Read the model definition and answer for the solid it produces. Units are mm, in the model's axes. A direction names the side the tool comes from. Round coordinates to 2 decimals unless told otherwise and drop trailing zeros. Write each loop counter-clockwise with the first axis right and the second up, starting at its lowest first coordinate (ties: lowest second). Pieces come first, ordered by that corner, then holes.
from build123d import *

# Parameters (mm, degrees)
SKETCH_1_R          = 3.05
EXTRUDE_1_DEPTH     = 12
SKETCH_2_R          = 3.098235282
EXTRUDE_2_DEPTH     = 2
EXTRUDE_3_DEPTH     = 7
CHAMFER_1_SIZE      = 1
SKETCH_6_R          = 3.05
CUT_EXTRUDE_2_DEPTH = 7
SKETCH_7_R          = 3.05
SKETCH_7_R_2        = 3
EXTRUDE_4_DEPTH     = 10
SKETCH_8_R          = 3
EXTRUDE_5_DEPTH     = 1


with BuildPart() as part:
    # 草图1 → 凸台-拉伸1 (new body)
    with BuildSketch(Plane.XY):
        Polygon((1.45714262, 6.138188374), (-2.429083459, 5.822385651), (-5.387482218, 3.282629506), (-6.288045884, -0.510979538), (-4.786789744, -4.109411766), (-1.45714262, -6.138188374), (2.429083459, -5.822385651), (5.387482218, -3.282629506), (6.288045884, 0.510979538), (4.786789744, 4.109411766), align=None)
        Circle(SKETCH_1_R, mode=Mode.SUBTRACT)
    extrude(amount=EXTRUDE_1_DEPTH)

    # 草图2 → 凸台-拉伸2 (add)
    with BuildSketch(Plane.XY.offset(12)):
        Circle(SKETCH_2_R)
    extrude(amount=-EXTRUDE_2_DEPTH)

    # 草图3 → 凸台-拉伸3 (add)
    with BuildSketch(Plane(origin=(0, 0, 10), x_dir=(-1, 0, 0), z_dir=(0, 0, -1))):
        with BuildLine():
            Line((1.45, 2.683281573), (1.45, -2.683281573))
            ThreePointArc((1.45, -2.683281573), (3.05, 0), (1.45, 2.683281573))
        make_face()
    extrude(amount=EXTRUDE_3_DEPTH)

    # 倒角1
    chamfer_1_edges = [part.edges().sort_by_distance(p)[0] for p in [
        (-3.908282839, 4.552507579, 12),
        (-5.837764051, 1.385824984, 12),
        (-5.537417814, -2.310195652, 12),
        (-3.121966182, -5.12380007, 12),
        (0.48597042, -5.980287012, 12),
        (3.908282839, -4.552507579, 12),
        (5.837764051, -1.385824984, 12),
        (5.537417814, 2.310195652, 12),
        (3.121966182, 5.12380007, 12),
        (-0.48597042, 5.980287012, 12),
    ]]
    chamfer(chamfer_1_edges, length=CHAMFER_1_SIZE)

    # 草图5 → 切除-放样1 section 0
    with BuildSketch(Plane.XY.offset(12)):
        Polygon((0.910714137, 3.836367733), (-1.518177162, 3.638991032), (-3.367176386, 2.051643441), (-3.930028677, -0.319362211), (-2.99174359, -2.568382354), (-0.910714137, -3.836367733), (1.518177162, -3.638991032), (3.367176386, -2.051643441), (3.930028677, 0.319362211), (2.99174359, 2.568382354), align=None)
    # 草图4 → 切除-放样1 section 1
    with BuildSketch(Plane.XY.offset(11)):
        Polygon((0.72857131, 3.069094187), (-1.21454173, 2.911192826), (-2.693741109, 1.641314753), (-3.144022942, -0.255489769), (-2.393394872, -2.054705883), (-0.72857131, -3.069094187), (1.21454173, -2.911192826), (2.693741109, -1.641314753), (3.144022942, 0.255489769), (2.393394872, 2.054705883), align=None)
    loft(mode=Mode.SUBTRACT)

    # 草图6 → 切除-拉伸2 (cut)
    with BuildSketch(Plane(origin=(0, 0, 3), x_dir=(-1, 0, 0), z_dir=(0, 0, -1))):
        Circle(SKETCH_6_R)
    extrude(amount=-CUT_EXTRUDE_2_DEPTH, mode=Mode.SUBTRACT)

    # 草图7 → 凸台-拉伸4 (add)
    with BuildSketch(Plane(origin=(0, 0, 0), x_dir=(-1, 0, 0), z_dir=(0, 0, -1))):
        Circle(SKETCH_7_R)
        Circle(SKETCH_7_R_2, mode=Mode.SUBTRACT)
    extrude(amount=-EXTRUDE_4_DEPTH)

    # 草图8 → 凸台-拉伸5 (add)
    with BuildSketch(Plane(origin=(0, 0, 0), x_dir=(-1, 0, 0), z_dir=(0, 0, -1))):
        Polygon((2.429083459, 5.822385651), (-1.45714262, 6.138188374), (-4.786789744, 4.109411766), (-6.288045884, 0.510979538), (-5.387482218, -3.282629506), (-2.429083459, -5.822385651), (1.45714262, -6.138188374), (4.786789744, -4.109411766), (6.288045884, -0.510979538), (5.387482218, 3.282629506), align=None)
        Circle(SKETCH_8_R, mode=Mode.SUBTRACT)
    extrude(amount=EXTRUDE_5_DEPTH)


solid = part.part
Q1. Determine the mould class of faces 3 (the cylindrical face through (3, 0, 5)), 4 (the flat face through (5.844, -1.359, 5.084)), 5 (the flat face through (-3.929, 4.535, 5.084)) for opening direction X: pulls with the +X half, pulls with the -X half, needs draft (parallel to the pull), parting line crosses it, or undercut.
Verdict:
face 3: undercut
face 4: pulls with the +X half
face 5: pulls with the -X half
Q2. Which of the six approach directions +Z, -Z, +X, -X, +Y, -Y give full straight-line access (tool end or side, diameter ignored) to faces 1 (the flat face through (5.093, 2.095, 11.493)), 2 (the flat face through (0, 0, 11))?
Verdict:
face 1: +Z, +X, +Y
face 2: +Z
Q3. Flat-ended cylindrical pins translate along their axes: pin 1 Ø5 at (x, z) = (-0.5, 2.5) entering from +Y; pin 2 Ø1 at (y, z) = (0, 8.5) entering from -X; pin 3 Ø1.8 at (x, y) = (-0.5, -0.5) entering from +Z; pin 4 Ø1.5 at (x, y) = (0.5, 3) entering from +Z. Find the tip coordinate at first contact, or state that the pin passes through.
Verdict:
pin 1: stops at y = 6.14
pin 2: stops at x = -6.29
pin 3: stops at z = 11
pin 4: stops at z = 11.93
Q4. Straight lines are drawn through the part: probe 1 along Z at (x, y) = (-1, 0.5); probe 2 along Y at (x, z) = (2, 7.5); probe 3 along Y at (x, z) = (2.75, 5). For each, find the intervals that lie inside material, in ascending order.
Verdict:
probe 1: z = 10 to 11
probe 2: y = -5.86 to -2.24, 2.24 to 5.81
probe 3: y = -5.55 to -1.2, 1.2 to 5.35
Q5. Section A-A (z = 8.75) is taken. Determine the outline of the cut face in (x, y), then the cut area to 3 significant figures.
Verdict:
outline: (-6.29, -0.51) - (-4.79, -4.11) - (-1.46, -6.14) - (2.43, -5.82) - (5.39, -3.28) - (6.29, 0.51) - (4.79, 4.11) - (1.46, 6.14) - (-2.43, 5.82) - (-5.39, 3.28) - close; hole circle Ø6 at (0, 0)
area: 88.7 mm2
